from build123d import *

# Parameters (mm, degrees)
ESQUISSE1_R          = 5
BASE_EXTRUSION_DEPTH = 2
ESQUISSE2_R          = 3
BOSS_EXTRU_1_DEPTH   = 10
CONG_1_R             = 2


with BuildPart() as part:
    # Esquisse1 → Base-Extrusion (new body)
    with BuildSketch(Plane.XY):
        Circle(ESQUISSE1_R)
    extrude(amount=BASE_EXTRUSION_DEPTH)

    # Esquisse2 → Boss.-Extru.1 (add)
    with BuildSketch(Plane.XY.offset(2)):
        Circle(ESQUISSE2_R)
    extrude(amount=BOSS_EXTRU_1_DEPTH)

    # Congé1
    cong_1_edges = [part.edges().sort_by_distance(p)[0] for p in [
        (-5, 0, 0),
    ]]
    fillet(cong_1_edges, radius=CONG_1_R - 0.0001)  # a hair under: the kernel refuses the full size


solid = part.part
Could you check a few things on this model? Use its own coordinates, in mm. A direction names the side the tool comes from. Give positions to 0.01 mm unless a question says otherwise; leave off trailing zeros. Order: outer loops, then holes, each group sorted by start corner. A loop starts at its lowest first (then second) coordinate and runs counter-clockwise, first axis right, second up. Notation, with made-up numbers: (56, -2) -> (73, -2) arc R16 cw to (73, 12) -> close; hole circle Ø9 at (16.25, 53). An arc over 180 degrees is marked (long way). Answer in a Markdown table with one row per item. Add a question column.
Item 1: Imagine slicing it at C-C (z = 5.25). List the corners of the cut face in (x, y) for me, and give its area (3 significant figures).
Item 2: Please list where these lines run through material, in increasing order: probe 1 along Z at (x, y) = (-3, -3.25); probe 2 along Y at (x, z) = (-1, 3.75); probe 3 along Z at (x, y) = (-2, -3.75).
Item 3: I'm going to push flat-ended pins straight in: P1, Ø6, axis at y = -3, z = 8, coming from the +X side; P2, Ø6, axis at y = -2, z = 1.5, coming from the +X side; P3, Ø2, axis at x = -3.5, y = 2.5, coming from the -Z side. Where does each tip first touch, or does it pass through?
Item 4: For faces 1 (the flat face through (-0.1, -3.3, 2)), 2 (the flat face through (0, 0, 12)), which set-ups out of +Z, -Z, +X, -X, +Y, -Y let a thin tool reach every point of the face, with its end or its side?
Result:
| question | item | result |
|---|---|---|
| 1 | outline | circle Ø6 at (0, 0) |
| 1 | area | 28.3 mm2 |
| 2 | probe 1 | 0.59 to 2 |
| 2 | probe 2 | -2.83 to 2.83 |
| 2 | probe 3 | 0.44 to 2 |
| 3 | P1 | x = 3 |
| 3 | P2 | x = 5 |
| 3 | P3 | z = 0.02 |
| 4 | face 1 | +Z |
| 4 | face 2 | +Z, +X, -X, +Y, -Y |
